Here's how the part is built. I have some questions about the finished solid (model axes, mm). A direction names the side the tool comes from. Round coordinates to 2 decimals unless told otherwise and drop trailing zeros. Write each loop counter-clockwise with the first axis right and the second up, starting at its lowest first coordinate (ties: lowest second). Pieces come first, ordered by that corner, then holes. Notation, with made-up numbers: M 49,-3.5 L 59,-3.5 A30 ccw 59,33.5 Z; hole C 76,81 d9. An arc over 180 degrees is marked long. Use a Markdown table: item, result. Add a question column.
```python
from build123d import *

# Parameters (mm, degrees)
SKETCH1_W           = 63.5
SKETCH1_H           = 12.7
SKETCH1_R           = 4.7625
BOSS_EXTRUDE1_DEPTH = 25.4
SKETCH2_R           = 1.9939
BOSS_EXTRUDE2_DEPTH = 19.05
SKETCH3_R           = 1.9939
BOSS_EXTRUDE3_DEPTH = 19.05


with BuildPart() as part:
    # Sketch1 → Boss-Extrude1 (new body)
    with BuildSketch(Plane.XY):
        Rectangle(SKETCH1_W, SKETCH1_H)
        Circle(SKETCH1_R, mode=Mode.SUBTRACT)
    extrude(amount=-BOSS_EXTRUDE1_DEPTH)

    # Sketch2 → Boss-Extrude2 (add)
    with BuildSketch(Plane(origin=(31.75, 0, 0), x_dir=(0, 0, -1), z_dir=(1, 0, 0))):
        with Locations((12.7, 0)):
            Circle(SKETCH2_R)
    extrude(amount=BOSS_EXTRUDE2_DEPTH)

    # Sketch3 → Boss-Extrude3 (add)
    with BuildSketch(Plane.ZY.offset(31.75)):
        with Locations((-12.7, 0)):
            Circle(SKETCH3_R)
    extrude(amount=BOSS_EXTRUDE3_DEPTH)


solid = part.part
```
Item 1: I need wall thicknesses on probe 1 along X at (y, z) = (0.25, -15.25); probe 2 along Y at (x, z) = (0, -17.25); probe 3 along X at (y, z) = (-5.5, -22). Which ranges of each line are inside material? Lowest first, please. Write a range as from..to.
Item 2: On a 3-axis mill with a long thin cutter (end or side, diameter ignored), from which of +Z, -Z, +X, -X, +Y, -Y can I reach the whole of each face in a straight line? I mean faces 1 (the face through (-41.1, 0.6, -10.8)), 2 (the face through (0, -6, 0)). Say none if no direction works.
Item 3: Imagine slicing it at B-B on y = 0. List the corners of the cut face in (x, z) for me, plus the area to 3 significant figures.
Item 4: Imagine slicing it at D-D on x = -35. List the corners of the cut face in (y, z) for me.
Item 5: Imagine slicing it at A-A on x = 0. List the corners of the cut face in (y, z) for me.
Item 6: For pin 1 Ø3 at (x, y) = (7, 4.5) entering from +Z; pin 2 Ø1.5 at (y, z) = (2.5, -4.5) entering from +X; pin 3 Ø3 at (x, z) = (-33.5, -10.5) entering from -Y; pin 4 Ø1 at (x, z) = (-38.5, -14.5) entering from +Y, each with a flat end and sliding along its axis, tell me the tip position at first contact or that it passes through.
Item 7: If we mould it in two halves opening along Y, with no side actions, what happens to faces 3 (the face through (-3.78, -2.9, -12.52)), 4 (the face through (-31.75, 0, -15)), 5 (the face through (41.14, 0.09, -10.71))? For each: +Y half, -Y half, draft (parallel to the pull), parting line (faces both ways), or undercut.
The answers:
| question | item | result |
|---|---|---|
| 1 | probe 1 | -31.75..-4.76, 4.76..31.75 |
| 1 | probe 2 | -6.35..-4.76, 4.76..6.35 |
| 1 | probe 3 | -31.75..31.75 |
| 2 | face 1 | -X |
| 2 | face 2 | +Z, +X, -X, +Y, -Y |
| 3 | outline | M -50.8,-14.69 L -31.75,-14.69 L -31.75,-25.4 L -4.76,-25.4 L -4.76,0 L -31.75,0 L -31.75,-10.71 L -50.8,-10.71 Z; M 4.76,-25.4 L 31.75,-25.4 L 31.75,-14.69 L 50.8,-14.69 L 50.8,-10.71 L 31.75,-10.71 L 31.75,0 L 4.76,0 Z |
| 3 | area | 1,520 mm² |
| 4 | outline | C 0,-12.7 d3.99 |
| 5 | outline | M -6.35,-25.4 L -4.76,-25.4 L -4.76,0 L -6.35,0 Z; M 4.76,-25.4 L 6.35,-25.4 L 6.35,0 L 4.76,0 Z |
| 6 | pin 1 | z = 0 |
| 6 | pin 2 | x = 31.75 |
| 6 | pin 3 | y = -1.87 |
| 6 | pin 4 | y = 1.51 |
| 7 | face 3 | undercut |
| 7 | face 4 | draft |
| 7 | face 5 | parting line |
